Autodesk Inventor part; units mm, degrees
ref_plane "YZ Plane" through (0, 0, 0) normal (1, 0, 0) x (0, 1, 0)
ref_plane "XZ Plane" through (0, 0, 0) normal (0, 1, 0) x (-1, 0, 0)
ref_plane "XY Plane" through (0, 0, 0) normal (0, 0, 1) x (1, 0, 0)
ref_plane "Arbeitsebene1" through (0.2798, 48.6, 0) normal (0, 0, 1) x (1, 0, 0)
ref_plane "Arbeitsebene2" through (106.3244, 12.4, 0) normal (0, 0, 1) x (-1, 0, 0)
sketch "Skizze8" plane through (106.3244, 12.4, 0) normal (0, 0, 1) x (-1, 0, 0)
  circle A0 centre (8.6702, 4) radius 1.4
  circle A1 centre (70.5201, 20.3) radius 1.4
  circle A2 centre (8.6702, 20.3) radius 1.4
  circle A3 centre (42.5201, 20.3) radius 1.4
  circle A4 centre (42.5201, 6.2) radius 1.4
  circle A5 centre (70.5201, 6.2) radius 1.4
  circle A6 centre (87.6702, 20.3) radius 1.4
  circle A7 centre (87.6702, 4) radius 1.4
  line L0 (5, 0) -> (5, 24.3)
  line L1 (5, 0) -> (90, 0)
  line L2 (90, 24.3) -> (90, 0)
  line L3 (26.35, 24.3) -> (90, 24.3)
  arc A8 (15.35, 24.3) -> (26.35, 24.3) centre (20.85, 24.3) ccw
  line L4 (5, 24.3) -> (15.35, 24.3)
  circle A9 centre (8.6702, 44.6) radius 1.4
  circle A10 centre (70.5201, 28.3) radius 1.4
  circle A11 centre (8.6702, 28.3) radius 1.4
  circle A12 centre (42.5201, 28.3) radius 1.4
  circle A13 centre (42.5201, 42.4) radius 1.4
  circle A14 centre (70.5201, 42.4) radius 1.4
  circle A15 centre (87.6702, 28.3) radius 1.4
  circle A16 centre (87.6702, 44.6) radius 1.4
  line L5 (5, 48.6) -> (5, 24.3)
  line L6 (5, 24.3) -> (15.35, 24.3)
  arc A17 (26.35, 24.3) -> (15.35, 24.3) centre (20.85, 24.3) ccw
  line L7 (26.35, 24.3) -> (90, 24.3)
  line L8 (90, 24.3) -> (90, 48.6)
  line L9 (5, 48.6) -> (90, 48.6)
  line L10 (8.1, 62.05) -> (8.1, -13.45)
  circle A18 centre (20.85, 24.3) radius 10
  line L11 (5, 0) -> (0, 0)
  line L12 (0, 0) -> (0, 48.6)
  line L13 (0, 48.6) -> (5, 48.6)
  line L14 (5, 48.6) -> (5, 0)
  point P0 (106.3244, 12.4)
  point P1 (8.1, 48.6)
  point P2 (8.1, 45.8786)
  point P3 (8.1, 43.3214)
  point P4 (8.1, 29.5786)
  point P5 (8.1, 27.0214)
  point P6 (8.1, 21.5786)
  point P7 (8.1, 19.0214)
  point P8 (8.1, 5.2786)
  point P9 (8.1, 2.7214)
  point P10 (8.1, 0)
  dimension "d36" = 20
  dimension "d38" = 5
extrude "Extrusion6" add sketch "Skizze8" along normal blind 10 contours A0 L10 | A0 L10 A2 L4 A18 L3 L2 L1 | L10 A0 | A0 L10 L1 L0 L4 A2 | L10 A2 | A2 L10 | L11 L12 L13 L5 L0 | L10 A11 A9 L9 L8 L3 A18 L4 | L4 L5 L9 L10 A9 A11 | L10 A11 | A11 L10 | L10 A9 | A9 L10
sketch "Skizze9" plane through (106.3244, 12.4, 10) normal (0, 0, 1) x (1, 0, 0)
  arc A0 (-23.35, -48.1544) -> (-18.35, -48.1544) centre (-20.85, -49.3) ccw
  line L0 (-23.35, -48.1544) -> (-23.35, -0.4456)
  arc A1 (-18.35, -0.4456) -> (-23.35, -0.4456) centre (-20.85, 0.7) ccw
  line L1 (-18.35, -0.4456) -> (-18.35, -48.1544)
  line L2 (-33.6, 13.45) -> (-33.6, -62.05)
  line L3 (-33.6, -62.05) -> (-8.1, -62.05)
  line L4 (-8.1, -62.05) -> (-8.1, 13.45)
  line L5 (-8.1, 13.45) -> (-33.6, 13.45)
  line L6 (-34.1, -62.55) -> (-34.1, 13.95)
  line L7 (-34.1, 13.95) -> (-7.6, 13.95)
  line L8 (-7.6, 13.95) -> (-7.6, -62.55)
  line L9 (-7.6, -62.55) -> (-34.1, -62.55)
  point P0 (-106.3244, -12.4)
  dimension "d37" = 0.5
extrude "Extrusion7" cut sketch "Skizze9" against normal blind 5 contours L0 A1 L1 A0 | L5 L4 L3 L2 | L6 L7 L8 L9
chamfer "Fasen2" distance 2 angle 45 6 edges at (72.2244, -11.9, 10) (98.7244, -11.9, 10) (16.3244, -36.2, 5) (16.3244, 12.4, 5) (106.3244, 12.4, 5) (106.3244, -36.2, 5)
sketch "Skizze10" plane through (106.3244, 12.4, 10) normal (0, 0, 1) x (1, 0, 0)
  circle A0 centre (-87.6702, -44.6) radius 1.4
  circle A1 centre (-70.5201, -42.4) radius 1.4
  circle A2 centre (-42.5201, -28.3) radius 1.4
  circle A3 centre (-70.5201, -28.3) radius 1.4
  circle A4 centre (-42.5201, -42.4) radius 1.4
  circle A5 centre (-87.6702, -28.3) radius 1.4
  circle A6 centre (-70.5201, -20.3) radius 1.4
  circle A7 centre (-42.5201, -20.3) radius 1.4
  circle A8 centre (-42.5201, -6.2) radius 1.4
  circle A9 centre (-70.5201, -6.2) radius 1.4
  circle A10 centre (-87.6702, -20.3) radius 1.4
  circle A11 centre (-87.6702, -4) radius 1.4
  line L0 (-36.1, 0) -> (-36.1, -48.6)
  line L1 (-36.1, 0) -> (-88, 0)
  line L2 (-90, -2) -> (-90, -46.6)
  line L3 (-88, -48.6) -> (-36.1, -48.6)
  line L4 (-90, -2) -> (-88, 0)
  line L5 (-88, -48.6) -> (-90, -46.6)
  line L6 (0, -46.6) -> (-2, -48.6)
  line L7 (0, -46.6) -> (0, -2)
  line L8 (-2, 0) -> (0, -2)
  line L9 (-2, 0) -> (-5.6, 0)
  line L10 (-5.6, -48.6) -> (-5.6, 0)
  line L11 (-5.6, -48.6) -> (-2, -48.6)
  point P0 (-106.3244, -12.4)
hole "Bohrung3" at (18.6542, 8.4, 10) at (18.6542, -7.9, 10) at (18.6542, -32.2, 10) at (18.6542, -15.9, 10) at (35.8043, -15.9, 10) at (35.8043, -7.9, 10) at (35.8043, -30, 10) at (63.8043, -30, 10) at (63.8043, -15.9, 10) at (63.8043, -7.9, 10) at (63.8043, 6.2, 10) at (35.8043, 6.2, 10) direction (0, 0, -1) diameter 3.6 depth 15 tip angle 118
sketch "Skizze11" plane through (106.3244, 12.4, 10) normal (0, 0, 1) x (1, 0, 0)
  point P0 (-106.3244, -12.4)
sketch "Skizze12" plane through (106.3244, 12.4, 10) normal (0, 0, 1) x (1, 0, 0)
  circle A0 centre (-70.5201, -6.2) radius 1.8
  circle A1 centre (-42.5201, -6.2) radius 1.8
  circle A2 centre (-42.5201, -20.3) radius 1.8
  circle A3 centre (-42.5201, -28.3) radius 1.8
  circle A4 centre (-42.5201, -42.4) radius 1.8
  circle A5 centre (-70.5201, -42.4) radius 1.8
  circle A6 centre (-70.5201, -20.3) radius 1.8
  circle A7 centre (-70.5201, -28.3) radius 1.8
  circle A8 centre (-87.6702, -28.3) radius 1.8
  circle A9 centre (-87.6702, -44.6) radius 1.8
  circle A10 centre (-87.6702, -20.3) radius 1.8
  circle A11 centre (-87.6702, -4) radius 1.8
  line L0 (-36.1, 0) -> (-36.1, -48.6)
  line L1 (-36.1, 0) -> (-88, 0)
  line L2 (-90, -2) -> (-90, -46.6)
  line L3 (-88, -48.6) -> (-36.1, -48.6)
  circle A12 centre (-20.85, -24.3) radius 10
  line L4 (-38.85, -38.3) -> (-2.85, -38.3)
  line L5 (-2.85, -38.3) -> (-2.85, -10.3)
  line L6 (-2.85, -10.3) -> (-38.85, -10.3)
  line L7 (-38.85, -10.3) -> (-38.85, -38.3)
  line L8 (-38.85, -38.3) -> (-2.85, -10.3) construction
  line L9 (-2.85, -38.3) -> (-38.85, -10.3) construction
  line L10 (-90, -2) -> (-88, 0)
  line L11 (-88, -48.6) -> (-90, -46.6)
  line L12 (0, -46.6) -> (-2, -48.6)
  line L13 (0, -46.6) -> (0, -2)
  line L14 (-2, 0) -> (0, -2)
  line L15 (-2, 0) -> (-5.6, 0)
  line L16 (-5.6, -48.6) -> (-5.6, 0)
  line L17 (-5.6, -48.6) -> (-2, -48.6)
  point P0 (-106.3244, -12.4)
  dimension "d51" = 36
  dimension "d52" = 28
hole "Bohrung4" at (67.4744, 2.1, 10) at (67.4744, -25.9, 10) at (103.4744, 2.1, 10) at (103.4744, -25.9, 10) direction (0, 0, -1) diameter 2.8 depth 15 tip angle 118
properties part number "60_Planktoscope_Sampleholder"
The listing builds one solid part. Answer for the finished solid, in the listing's coordinates (mm). A direction names the side the tool comes from. Give positions to 0.01 mm unless a question says otherwise; leave off trailing zeros. Order: outer loops, then holes, each group sorted by start corner. A loop starts at its lowest first (then second) coordinate and runs counter-clockwise, first axis right, second up. Notation, with made-up numbers: (29, 57) -> (40, 57) arc R24 ccw to (40, 92) -> close; hole circle Ø9 at (-12, 30). An arc over 180 degrees is marked (long way). Put each result on its own line as item: value.
Item 1: Straight lines are drawn through the part: line 1 (X direction, y = -25.9, z = 3); line 2 (X direction, y = -5.5, z = 7); line 3 (Y direction, x = 37, z = 9.5). For each, find the intervals that lie inside material, in ascending order.
Established:
line 1: x = 16.32 to 66.07, 68.87 to 102.07, 104.87 to 106.32
line 2: x = 16.32 to 72.22, 98.72 to 106.32
line 3: y = -36.2 to -31.35, -28.65 to -17.25, -14.55 to -9.25, -6.55 to 4.85, 7.55 to 12.4
Item 2: For faces 4 (the face through (72.224, -12, 7)), 5 (the face through (37.56, -15.51, 4.93)), determine the directions among +Z, -Z, +X, -X, +Y, -Y from which every point of the face is accessible in a straight line to the end or side of a thin tool.
Established:
face 4: +Z, +Y, -Y
face 5: +Z, -Z
Item 3: For a pull along X with two mould halves and no side action, classify faces 1 (the face through (62, 12.4, 5)), 2 (the face through (16.324, -12, 5)), 3 (the face through (104.84, -25.6, 4.93)) as released by +X, released by -X, zero draft, split by the parting line, or undercut.
Established:
face 1: zero draft
face 2: released by -X
face 3: undercut
Item 4: A cutting plane is placed at C-C on y = -15. Give the vertices of the cut face in (x, z).
Established:
outline: (16.32, 0) -> (17.1, 0) -> (17.1, 10) -> (16.32, 10) -> close; (20.21, 0) -> (34.25, 0) -> (34.25, 10) -> (20.21, 10) -> close; (37.36, 0) -> (62.25, 0) -> (62.25, 10) -> (37.36, 10) -> close; (65.36, 0) -> (75.97, 0) -> (75.97, 5) -> (72.22, 5) -> (72.22, 8) -> (70.22, 10) -> (65.36, 10) -> close; (94.98, 0) -> (106.32, 0) -> (106.32, 10) -> (100.72, 10) -> (98.72, 8) -> (98.72, 5) -> (94.98, 5) -> close
Item 5: A cutting plane is placed at B-B on x = 89.5. Give the vertices of the cut face in (y, z), plus the area to 3 significant figures.
Established:
outline: (-36.2, 0) -> (-21.05, 0) -> (-21.05, 5) -> (-36.2, 5) -> close; (-2.75, 0) -> (12.4, 0) -> (12.4, 5) -> (-2.75, 5) -> close
area: 151 mm^2
Item 6: A cutting plane is placed at D-D on z = 6.75. Count the separate pieces of the cut face and the enclosed holes in it, plus the area to 3 significant figures.
Established:
separate pieces: 2
enclosed holes: 16
area: 2,930 mm^2
Item 7: Given P1, Ø3, axis at x = 35.8, y = -30, coming from the -Z side, flat-ended and moving along its own axis, determine where the tip first touches the part or whether it passes through.
Established:
P1: passes through
Item 8: A cutting plane is placed at A-A on y = -25.9. Give the vertices of the cut face in (x, z).
Established:
outline: (16.32, 0) -> (66.07, 0) -> (66.07, 10) -> (16.32, 10) -> close; (68.87, 0) -> (102.07, 0) -> (102.07, 10) -> (100.72, 10) -> (98.72, 8) -> (98.72, 5) -> (72.22, 5) -> (72.22, 8) -> (70.22, 10) -> (68.87, 10) -> close; (104.87, 0) -> (106.32, 0) -> (106.32, 10) -> (104.87, 10) -> close
